Could you check a few things on this drawing? It's one solid part, dimensions in mm from its lowest x, y, z. A direction names the side the tool comes from. Round coordinates to 2 decimals unless told otherwise and drop trailing zeros. Write each loop counter-clockwise with the first axis right and the second up, starting at its lowest first coordinate (ties: lowest second). Pieces come first, ordered by that corner, then holes. Notation, with made-up numbers: (-19, -35.75) -> (6, -35.75) arc R10 ccw to (6, -19.75) -> close; hole circle Ø10 at (48, 76). An arc over 180 degrees is marked (long way). Answer as CSV lines item,"result".
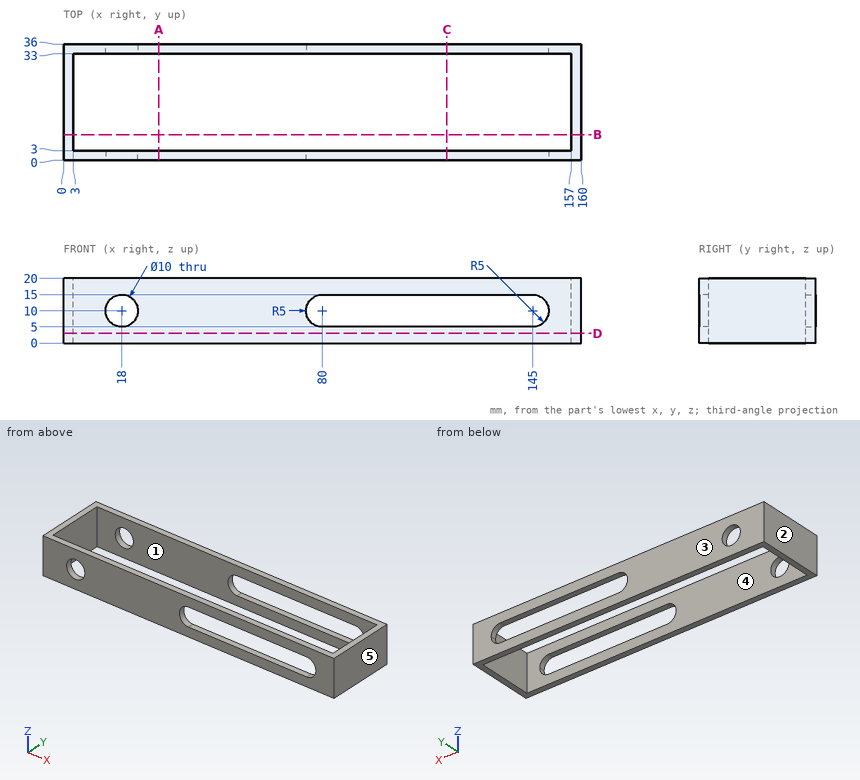
1. Suppose I cut it at D-D on z = 3. Please give me the cut outline in (x, y), and give its area (3 significant figures).
Numbers:
outline,"(0, 0) -> (160, 0) -> (160, 36) -> (0, 36) -> close; hole (3, 3) -> (157, 3) -> (157, 33) -> (3, 33) -> close"
area,"1,140 mm^2"
2. Suppose I cut it at C-C on x = 118.5. Please give me the cut outline in (y, z), and give its area (3 significant figures).
Numbers:
outline,"(0, 0) -> (3, 0) -> (3, 5) -> (0, 5) -> close; (0, 15) -> (3, 15) -> (3, 20) -> (0, 20) -> close; (33, 0) -> (36, 0) -> (36, 5) -> (33, 5) -> close; (33, 15) -> (36, 15) -> (36, 20) -> (33, 20) -> close"
area,"60.0 mm^2"
3. If I drill on line 1 (Y direction, x = 9, z = 14); line 2 (X direction, y = 7.5, z = 16.5); line 3 (Z direction, x = 18, y = 35), over which ranges is the centre line in solid material (lowest first)?
Numbers:
line 1,"y = 0 to 3, 33 to 36"
line 2,"x = 0 to 3, 157 to 160"
line 3,"z = 0 to 5, 15 to 20"
4. Suppose I cut it at B-B on y = 8. Please give me the cut outline in (x, z).
Numbers:
outline,"(0, 0) -> (3, 0) -> (3, 20) -> (0, 20) -> close; (157, 0) -> (160, 0) -> (160, 20) -> (157, 20) -> close"
5. Suppose I cut it at A-A on x = 29.5. Please give me the cut outline in (y, z), and give its area (3 significant figures).
Numbers:
outline,"(0, 0) -> (3, 0) -> (3, 20) -> (0, 20) -> close; (33, 0) -> (36, 0) -> (36, 20) -> (33, 20) -> close"
area,"120 mm^2"
6. On a 3-axis mill with a long thin cutter (end or side, diameter ignored), from which of +Z, -Z, +X, -X, +Y, -Y can I reach the whole of each face in a straight line? I mean the marked faces 1 and 2. Say none if no direction works.
Numbers:
face 1,"+Z, -Z"
face 2,"+Z, -Z, -X, +Y, -Y"
7. For pin 1 Ø2 at (x, z) = (141.5, 17.5) entering from -Y, with a flat end and sliding along its axis, tell me the tip position at first contact or that it passes through.
Numbers:
pin 1,"stops at y = 0"
8. If we mould it in two halves opening along X, with no side actions, what happens to the marked faces 3, 4 and 5? For each: released by +X, released by -X, zero draft, split by the parting line, or undercut.
Numbers:
face 3,"zero draft"
face 4,"undercut"
face 5,"released by +X"
